Autodesk Inventor part; units mm, degrees
ref_plane "Arbeitsebene1" through (0, 3, 0) normal (0, 1, 0) x (-1, 0, 0)
ref_plane "YZ Plane" through (0, 0, 0) normal (1, 0, 0) x (0, 1, 0)
ref_plane "XY Plane" through (0, 0, 0) normal (0, 0, 1) x (1, 0, 0)
sketch "Skizze1" plane through (0, 0, 0) normal (0, 1, 0) x (-1, 0, 0)
  line L0 (0, 0) -> (2, 0)
  line L1 (2, 0) -> (2, -10)
  line L2 (2, -10) -> (3, -10)
  line L3 (3, -10) -> (3, -71)
  line L4 (3, -71) -> (2, -71)
  line L5 (2, -71) -> (2, -93)
  line L6 (2, -93) -> (0, -93)
  line L7 (0, -93) -> (0, 0)
  dimension "d0" = 10
  dimension "d1" = 22
  dimension "d2" = 93
  dimension "d3" = 4
  dimension "d4" = 6
revolve "Umdrehung1" add sketch "Skizze1" angle 360 about axis through (0, 0, -93) along (0, 0, 1)
thread "Gewinde1"
ref_plane "Arbeitsebene1" through (0, 3, 0) normal (0, 1, 0) x (-1, 0, 0)
sketch "Skizze2" plane through (0, 3, 0) normal (0, 1, 0) x (-1, 0, 0)
  line L0 (3, -10) -> (-3, -10)
  line L1 (3, -71) -> (-3, -71)
  point P0 (0, 0)
  point P1 (0, -61)
  dimension "d9" = 10
hole "Bohrung1" at (0, 3, -61) direction (0, -1, 0) diameter 2.5 end through all
chamfer "Fasen1" distance 0.5 angle 45 1 edges at (2, 0, -93)
properties part number "205 part 1" material "Aluminium 6061"
Can you work these out from the model? Positions are in its coordinate system, mm. A direction names the side the tool comes from. Round coordinates to 2 decimals unless told otherwise and drop trailing zeros. Loops run counter-clockwise (first coordinate to the right, second up) from the corner with the lowest first, then second, coordinate; pieces in that order, holes last. Notation, with made-up numbers: (54.5, -17.5) -> (77.5, -17.5) arc R15 cw to (77.5, -6.5) -> close; hole circle Ø6 at (-33, 16). An arc over 180 degrees is marked (long way). One line per item, written item: value. Start each with the question number.
1. If we section it at C-C, the plane z = -21.5: Write out the boundary of the cut face in (x, y), then the cut area to 3 significant figures.
2. If we section it at D-D, the plane z = -61: Write out the boundary of the cut face in (x, y), then the cut area to 3 significant figures.
3. If we mould it in two halves opening along Z, with no side actions, what happens to faces 4 (the cylindrical face through (-0.38, -0.04, -59.81)), 5 (the flat face through (0, 0, -93)), 6 (the cylindrical face through (0, -2, -82)), 7 (the flat face through (-1, 2, -10))? For each: pulls with the +Z half, pulls with the -Z half, needs draft (parallel to the pull), parting line crosses it, or undercut.
4. If we section it at B-B, the plane y = 0: Write out the boundary of the cut face in (x, z).
5. If we section it at A-A, the plane x = 0: Write out the boundary of the cut face in (y, z).
6. For pin 1 (1.5 mm diameter, centred on y = 2.5, z = -73.5, fed in from -X); pin 2 (3 mm diameter, centred on x = 1.5, z = -59.5, fed in from +Y); pin 3 (1 mm diameter, centred on x = 2.5, z = -10, fed in from +Y); pin 4 (1 mm diameter, centred on y = 1.5, z = -69.5, fed in from +X), each with a flat end and sliding along its axis, tell me the tip position at first contact or that it passes through.
7. For faces 1 (the flat face through (0, 0, 0)), 2 (the flat face through (-1, 2, -71)), 3 (the cylindrical face through (0, -2, -5)), which set-ups out of +Z, -Z, +X, -X, +Y, -Y let a thin tool reach every point of the face, with its end or its side?
8. If I drill on probe 1 along Z at (x, y) = (0, 0); probe 2 along X at (y, z) = (-0.25, -61); probe 3 along X at (y, z) = (1.25, -61), over which ranges is the centre line in solid material (lowest first)?
Calculated:
1. outline: circle Ø6 at (0, 0)
1. area: 28.3 mm²
2. outline: (-1.25, -2.73) -> (-1.25, 2.73) arc R3 ccw to start; (1.25, -2.73) arc R3 ccw to (1.25, 2.73) -> close
2. area: 13.7 mm²
3. face 4: undercut
3. face 5: pulls with the -Z half
3. face 6: needs draft
3. face 7: pulls with the +Z half
4. outline: (-3, -71) -> (-2, -71) -> (-2, -92.5) -> (-1.5, -93) -> (1.5, -93) -> (2, -92.5) -> (2, -71) -> (3, -71) -> (3, -10) -> (2, -10) -> (2, 0) -> (-2, 0) -> (-2, -10) -> (-3, -10) -> close; hole circle Ø2.5 at (0, -61)
5. outline: (-3, -71) -> (-2, -71) -> (-2, -92.5) -> (-1.5, -93) -> (1.5, -93) -> (2, -92.5) -> (2, -71) -> (3, -71) -> (3, -62.25) -> (-3, -62.25) -> close; (-3, -59.75) -> (3, -59.75) -> (3, -10) -> (2, -10) -> (2, 0) -> (-2, 0) -> (-2, -10) -> (-3, -10) -> close
6. pin 1: stops at x = -0.97
6. pin 2: stops at y = 3
6. pin 3: stops at y = 2.24
6. pin 4: stops at x = 2.83
7. face 1: +Z, +X, -X, +Y, -Y
7. face 2: -Z
7. face 3: +Z
8. probe 1: z = -93 to -62.25, -59.75 to 0
8. probe 2: x = -2.99 to -1.25, 1.25 to 2.99
8. probe 3: x = -2.73 to -1.25, 1.25 to 2.73
